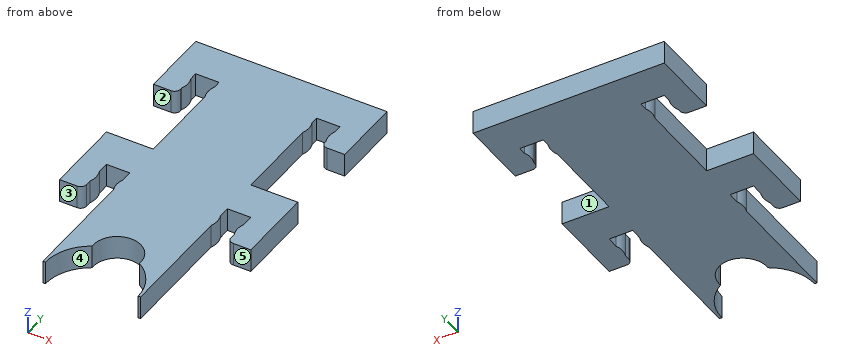
```python
from build123d import *

# Parameters (mm, degrees)
BOSS_EXTRUDE1_DEPTH = 3
FILLET1_R           = 0.75


with BuildPart() as part:
    # Sketch1 → Boss-Extrude1 (new body)
    with BuildSketch(Plane.XY):
        with BuildLine():
            Line((12.840070534, 24.147116385), (-11.659929466, 24.147116385))
            Line((-11.659929466, 24.147116385), (-11.659929466, 15.147116385))
            Line((-11.659929466, 15.147116385), (-8.659929466, 15.147116385))
            Line((-8.659929466, 15.147116385), (-8.659929466, 16.147116385))
            ThreePointArc((-8.659929466, 16.147116385), (-8.459929466, 17.147116385), (-8.659929466, 18.147116385))
            Line((-8.659929466, 18.147116385), (-8.659929466, 19.147116385))
            Line((-8.659929466, 19.147116385), (-5.659929466, 19.147116385))
            Line((-5.659929466, 19.147116385), (-5.659929466, 18.147116385))
            ThreePointArc((-5.659929466, 18.147116385), (-5.859929466, 17.147116385), (-5.659929466, 16.147116385))
            Line((-5.659929466, 16.147116385), (-5.659929466, 5.147116385))
            Line((-5.659929466, 5.147116385), (-11.659929466, 5.147116385))
            Line((-11.659929466, 5.147116385), (-11.659929466, -4.852883615))
            Line((-11.659929466, -4.852883615), (-8.659929466, -4.852883615))
            Line((-8.659929466, -4.852883615), (-8.659929466, -3.352883615))
            ThreePointArc((-8.659929466, -3.352883615), (-8.459929466, -2.352883615), (-8.659929466, -1.352883615))
            Line((-8.659929466, -1.352883615), (-8.659929466, 0.147116385))
            Line((-8.659929466, 0.147116385), (-5.659929466, 0.147116385))
            Line((-5.659929466, 0.147116385), (-5.659929466, -1.352883615))
            ThreePointArc((-5.659929466, -1.352883615), (-5.859929466, -2.352883615), (-5.659929466, -3.352883615))
            Line((-5.659929466, -3.352883615), (-5.659929466, -18.352883615))
            Line((-5.659929466, -18.352883615), (-5.344929466, -18.352883615))
            ThreePointArc((-5.344929466, -18.352883615), (-4.566833019, -15.415100311), (-2.436565272, -13.247621556))
            ThreePointArc((-2.436565272, -13.247621556), (0.447544838, -9.926226501), (3.630070534, -12.962883615))
            ThreePointArc((3.630070534, -12.962883615), (3.626727648, -13.105409311), (3.616706341, -13.247621556))
            ThreePointArc((3.616706341, -13.247621556), (5.746974087, -15.415100311), (6.525070534, -18.352883615))
            Line((6.525070534, -18.352883615), (6.840070534, -18.352883615))
            Line((6.840070534, -18.352883615), (6.840070534, -3.352883615))
            ThreePointArc((6.840070534, -3.352883615), (7.040070534, -2.352883615), (6.840070534, -1.352883615))
            Line((6.840070534, -1.352883615), (6.840070534, 0.147116385))
            Line((6.840070534, 0.147116385), (9.840070534, 0.147116385))
            Line((9.840070534, 0.147116385), (9.840070534, -1.352883615))
            ThreePointArc((9.840070534, -1.352883615), (9.640070534, -2.352883615), (9.840070534, -3.352883615))
            Line((9.840070534, -3.352883615), (9.840070534, -4.852883615))
            Line((9.840070534, -4.852883615), (12.840070534, -4.852883615))
            Line((12.840070534, -4.852883615), (12.840070534, 5.147116385))
            Line((12.840070534, 5.147116385), (6.840070534, 5.147116385))
            Line((6.840070534, 5.147116385), (6.840070534, 16.147116385))
            ThreePointArc((6.840070534, 16.147116385), (7.040070534, 17.147116385), (6.840070534, 18.147116385))
            Line((6.840070534, 18.147116385), (6.840070534, 19.147116385))
            Line((6.840070534, 19.147116385), (9.840070534, 19.147116385))
            Line((9.840070534, 19.147116385), (9.840070534, 18.147116385))
            ThreePointArc((9.840070534, 18.147116385), (9.640070534, 17.147116385), (9.840070534, 16.147116385))
            Line((9.840070534, 16.147116385), (9.840070534, 15.147116385))
            Line((9.840070534, 15.147116385), (12.840070534, 15.147116385))
            Line((12.840070534, 15.147116385), (12.840070534, 24.147116385))
        make_face()
    extrude(amount=BOSS_EXTRUDE1_DEPTH)

    # Fillet1
    fillet1_edges = [part.edges().sort_by_distance(p)[0] for p in [
        (-8.659929466, 15.147116385, 1.5),
        (9.840070534, 15.147116385, 1.5),
        (9.840070534, -4.852883615, 1.5),
        (-8.659929466, -4.852883615, 1.5),
    ]]
    fillet(fillet1_edges, radius=FILLET1_R)


solid = part.part
```
The model under review builds one solid part; all positions refer to its coordinate system, in mm. Face numbers are marked on the shaded views. A direction names the side the tool comes from. Coordinates: 2 decimals unless noted, no trailing zeros. Write each loop counter-clockwise with the first axis right and the second up, starting at its lowest first coordinate (ties: lowest second). Pieces come first, ordered by that corner, then holes.
1) We need section D-D on x = 1.25. State the section outline as (y, z) points, then the cut area to 3 significant figures.
2) To check wall thickness, follow probe 1 along X at (y, z) = (16, 1.2); probe 2 along X at (y, z) = (17, 0.8); probe 3 along Y at (x, z) = (-8, 1.6). State the ranges of each line that lie inside material, in increasing order.
3) We need section B-B on y = -11. State the section outline as (x, z) points.
4) Machinability: for the marked faces 1, 2 and 3, which of the approach directions +Z, -Z, +X, -X, +Y, -Y give a long, thin tool a straight path to every point of the face, cutting with its end or side? Answer none if there is none.
5) Clearance check with flat-ended pins moving along their axes: pin 1 Ø1.1 at (x, z) = (-10, 2) entering from -Y; pin 2 Ø0.9 at (x, z) = (-6.5, 2) entering from -Y. State where each tip first meets the part, or that it passes through.
6) We need section A-A on x = 7.75. State the section outline as (y, z) points, then the cut area to 3 significant figures.
7) We need section C-C on y = -2. State the section outline as (x, z) points, then the cut area to 3 significant figures.
8) The part is to be moulded in two halves that separate along X. For the marked faces 4 and 5, say which applies: pulls with the +X half, pulls with the -X half, needs draft (parallel to the pull), parting line crosses it, or undercut.
Answer list:
1. outline: (-10, 0) - (24.15, 0) - (24.15, 3) - (-10, 3) - close
1. area: 102 mm2
2. probe 1: x = -11.66 to -8.66, -5.66 to 6.84, 9.84 to 12.84
2. probe 2: x = -11.66 to -8.46, -5.86 to 7.04, 9.64 to 12.84
2. probe 3: y = 0.15 to 5.15, 19.15 to 24.15
3. outline: (-5.66, 0) - (-1.73, 0) - (-1.73, 3) - (-5.66, 3) - close; (2.91, 0) - (6.84, 0) - (6.84, 3) - (2.91, 3) - close
4. face 1: +Z, -Z, +X
4. face 2: +Z, -Z, -X
4. face 3: +Z, -Z, -X, -Y
5. pin 1: stops at y = -4.85
5. pin 2: stops at y = 0.15
6. outline: (0.15, 0) - (5.15, 0) - (5.15, 3) - (0.15, 3) - close; (19.15, 0) - (24.15, 0) - (24.15, 3) - (19.15, 3) - close
6. area: 30.0 mm2
7. outline: (-11.66, 0) - (-8.48, 0) - (-8.48, 3) - (-11.66, 3) - close; (-5.84, 0) - (7.02, 0) - (7.02, 3) - (-5.84, 3) - close; (9.66, 0) - (12.84, 0) - (12.84, 3) - (9.66, 3) - close
7. area: 57.6 mm2
8. face 4: undercut
8. face 5: needs draft
